The listing builds one solid part. Answer for the finished solid, in the listing's coordinates (mm). Face numbers are marked on the shaded views. A direction names the side the tool comes from. Give positions to 0.01 mm unless a question says otherwise; leave off trailing zeros. Write each loop counter-clockwise with the first axis right and the second up, starting at its lowest first coordinate (ties: lowest second). Pieces come first, ordered by that corner, then holes. Notation, with made-up numbers: (-34, -24.5) - (-16, -24.5) arc R16 cw to (-16, -18.5) - close; hole circle Ø9 at (85.25, -16). An arc over 180 degrees is marked (long way). One line per question, with ' | ' between items. Start each with the question number.
1. Find the intervals of material crossed by L1, parallel to Z at x = 15, y = 2.2; L2, parallel to X at y = 1.9, z = 44; L3, parallel to Y at x = 14, z = 18.5, in increasing order. Write a range as from..to.
2. Given P1, Ø12, axis at x = 7, z = 38.5, coming from the -Y side; P2, Ø4, axis at x = 15, z = 44, coming from the -Y side; P3, Ø4, axis at y = 23, z = 21, coming from the +X side, each flat-ended and moving along its own axis, determine where each tip first touches the part or whether it passes through.
3. For the marked faces 1 and 2, determine the directions among +Z, -Z, +X, -X, +Y, -Y from which every point of the face is accessible in a straight line to the end or side of a thin tool.
4. A cutting plane is placed at D-D (y = 2). Determine the outline of the cut face in (x, z).
5. A cutting plane is placed at C-C (z = 7). Determine the outline of the cut face in (x, y).
6. A cutting plane is placed at B-B (x = 15). Determine the outline of the cut face in (y, z), then the cut area to 3 significant figures.
7. A cutting plane is placed at A-A (y = 15). Determine the outline of the cut face in (x, z).
```python
from build123d import *

# Parameters (mm, degrees)
BOSS_EXTRUDE1_DEPTH      = 60
M6_CLEARANCE_HOLE1_D     = 6.4
M6_CLEARANCE_HOLE1_DEPTH = 8
M6_CLEARANCE_HOLE1_TIP   = 1.922753981
M5_CLEARANCE_HOLE1_D     = 5.3
M5_CLEARANCE_HOLE1_DEPTH = 8
M5_CLEARANCE_HOLE1_TIP   = 1.59228064


with BuildPart() as part:
    # Sketch1 → Boss-Extrude1 (new body)
    with BuildSketch(Plane.XY):
        Polygon((0, 30), (0, 0), (30, 0), (30, 4), (4, 4), (4, 30), align=None)
    extrude(amount=BOSS_EXTRUDE1_DEPTH)

    # M6 Clearance Hole1
    with Locations(Plane.ZY):
        with Locations((7, 15), (53, 15)):
            Hole(M6_CLEARANCE_HOLE1_D / 2, depth=M6_CLEARANCE_HOLE1_DEPTH)
            with Locations((0, 0, -(M6_CLEARANCE_HOLE1_DEPTH + M6_CLEARANCE_HOLE1_TIP / 2))):  # 118° drill point
                Cone(0, M6_CLEARANCE_HOLE1_D / 2, M6_CLEARANCE_HOLE1_TIP, mode=Mode.SUBTRACT)

    # M5 Clearance Hole1
    with Locations(Plane(origin=(0, 0, 0), x_dir=(-1, 0, 0), z_dir=(0, -1, 0))):
        with Locations((-15, -16), (-15, -44)):
            Hole(M5_CLEARANCE_HOLE1_D / 2, depth=M5_CLEARANCE_HOLE1_DEPTH)
            with Locations((0, 0, -(M5_CLEARANCE_HOLE1_DEPTH + M5_CLEARANCE_HOLE1_TIP / 2))):  # 118° drill point
                Cone(0, M5_CLEARANCE_HOLE1_D / 2, M5_CLEARANCE_HOLE1_TIP, mode=Mode.SUBTRACT)


solid = part.part
```
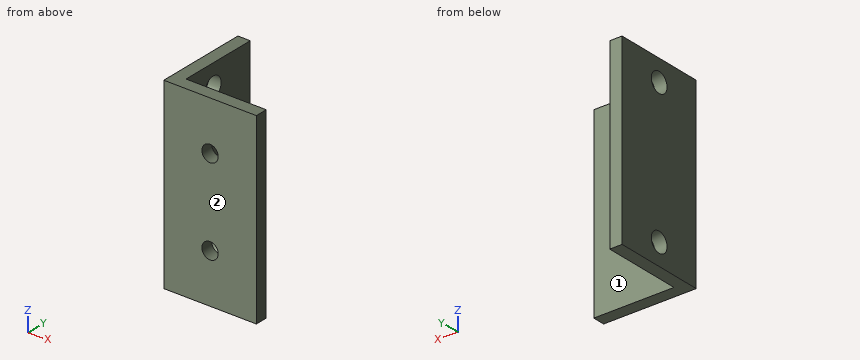
Determined:
1) L1: 0..13.35, 18.65..41.35, 46.65..60 | L2: 0..12.35, 17.65..30 | L3: 0..4
2) P1: y = 0 | P2: through | P3: x = 4
3) face 1: +Z, -Z, +X, +Y | face 2: +Z, -Z, +X, -X, -Y
4) outline: (0, 0) - (30, 0) - (30, 60) - (0, 60) - close; hole circle Ø5.3 at (15, 16); hole circle Ø5.3 at (15, 44)
5) outline: (0, 0) - (30, 0) - (30, 4) - (4, 4) - (4, 11.8) - (0, 11.8) - close; (0, 18.2) - (4, 18.2) - (4, 30) - (0, 30) - close
6) outline: (0, 0) - (4, 0) - (4, 13.35) - (0, 13.35) - close; (0, 18.65) - (4, 18.65) - (4, 41.35) - (0, 41.35) - close; (0, 46.65) - (4, 46.65) - (4, 60) - (0, 60) - close | area: 198 mm2
7) outline: (0, 0) - (4, 0) - (4, 3.8) - (0, 3.8) - close; (0, 10.2) - (4, 10.2) - (4, 49.8) - (0, 49.8) - close; (0, 56.2) - (4, 56.2) - (4, 60) - (0, 60) - close
